from build123d import *

# Parameters (mm, degrees)
F0_W     = 114.3
F0_H     = 330.2
F1_DEPTH = 5.842
F2_W     = 38.1
F2_H     = 5.842
F2_W_2   = 5.842
F2_H_2   = 25.4
F3_DEPTH = 25.4
F4_R     = 9.525
F5_DEPTH = 5.842


# Not quite as in the source:
# - a feature names something its author has since deleted; it is built from what else it names


with BuildPart() as f1:
    # F0 (on Front) → F1 (new body)
    with BuildSketch(Plane.XZ):
        with Locations((-25.4490938969, 91.3394362139)):
            Rectangle(F0_W, F0_H)
    extrude(amount=F1_DEPTH)

    # F2 (on face) → F3 (cut)
    with BuildSketch(Plane.XZ.offset(5.842)):
        Polygon((-82.5990938969, -73.7605637861), (-69.8990938969, -73.7605637861), (-69.8990938969, -67.9185637861), (-76.7570938969, -67.9185637861), (-76.7570938969, -48.3605637861), (-82.5990938969, -48.3605637861), align=None)
        with Locations((-25.4490938969, -70.8395637861)):
            Rectangle(F2_W, F2_H)
        Polygon((19.0009061031, -67.9185637861), (19.0009061031, -73.7605637861), (31.7009061031, -73.7605637861), (31.7009061031, -48.3605637861), (25.8589061031, -48.3605637861), (25.8589061031, -67.9185637861), align=None)
        with Locations((-79.6780938969, -10.2605637861)):
            Rectangle(F2_W_2, F2_H_2)
        with Locations((28.7799061031, -10.2605637861)):
            Rectangle(F2_W_2, F2_H_2)
        with Locations((-79.6780938969, 40.5394362139)):
            Rectangle(F2_W_2, F2_H_2)
        with Locations((28.7799061031, 40.5394362139)):
            Rectangle(F2_W_2, F2_H_2)
        with Locations((-79.6780938969, 91.3394362139)):
            Rectangle(F2_W_2, F2_H_2)
        with Locations((28.7799061031, 91.3394362139)):
            Rectangle(F2_W_2, F2_H_2)
        with Locations((-79.6780938969, 142.1394362139)):
            Rectangle(F2_W_2, F2_H_2)
        with Locations((28.7799061031, 142.1394362139)):
            Rectangle(F2_W_2, F2_H_2)
        with Locations((-79.6780938969, 192.9394362139)):
            Rectangle(F2_W_2, F2_H_2)
        with Locations((28.7799061031, 192.9394362139)):
            Rectangle(F2_W_2, F2_H_2)
        with Locations((28.7799061031, 243.7394362139)):
            Rectangle(F2_W_2, F2_H_2)
        with Locations((-79.6780938969, 243.7394362139)):
            Rectangle(F2_W_2, F2_H_2)
    extrude(amount=-F3_DEPTH, mode=Mode.SUBTRACT)

    # F4 (on face) → F5 (cut, through all)
    with BuildSketch(Plane.XZ.offset(5.842)):
        with BuildLine():
            ThreePointArc((-11.7009406501, 159.6019361475), (-10.1150214145, 163.4306838358), (-9.5740938969, 167.5394362139))
            ThreePointArc((-9.5740938969, 167.5394362139), (-10.1150214004, 171.6481885393), (-11.7009405957, 175.4769361859))
            ThreePointArc((-11.7009405957, 175.4769361859), (-17.5115938829, 181.2875894909), (-25.4490938969, 183.4144362139))
            ThreePointArc((-25.4490938969, 183.4144362139), (-33.3865937403, 181.2875895894), (-39.1972470011, 175.4769365272))
            ThreePointArc((-39.1972470011, 175.4769365272), (-41.3240938969, 167.5394362139), (-39.1972470011, 159.6019359006))
            ThreePointArc((-39.1972470011, 159.6019359006), (-33.3865937403, 153.7912828383), (-25.4490938969, 151.6644362139))
            ThreePointArc((-25.4490938969, 151.6644362139), (-17.5115939301, 153.7912829096), (-11.7009406501, 159.6019361475))
        make_face()
        with Locations((-57.1990938969, 243.7394362139)):
            Circle(F4_R)
        with Locations((6.3009061031, 243.7394362139)):
            Circle(F4_R)
        Polygon((-32.5182228501, 91.3394362139), (-41.6836583735, 107.2144362139), (-60.0145294203, 107.2144362139), (-69.1799649437, 91.3394362139), (-60.0145294203, 75.4644362139), (-41.6836583735, 75.4644362139), align=None)
        Polygon((18.2817771499, 91.3394362139), (9.1163416265, 107.2144362139), (-9.2145294203, 107.2144362139), (-18.3799649437, 91.3394362139), (-9.2145294203, 75.4644362139), (9.1163416265, 75.4644362139), align=None)
        with BuildLine():
            ThreePointArc((-39.1972470011, 175.4769365272), (-33.3865937403, 181.2875895894), (-25.4490938969, 183.4144362139))
            Line((-25.4490938969, 183.4144362139), (-34.6145294203, 183.4144362139))
            Line((-34.6145294203, 183.4144362139), (-39.1972470011, 175.4769365272))
        make_face()
        with BuildLine():
            ThreePointArc((-25.4490938969, 183.4144362139), (-17.5115938829, 181.2875894909), (-11.7009405957, 175.4769361859))
            Line((-11.7009405957, 175.4769361859), (-16.2836583735, 183.4144362139))
            Line((-16.2836583735, 183.4144362139), (-25.4490938969, 183.4144362139))
        make_face()
        with BuildLine():
            ThreePointArc((-11.7009405957, 175.4769361859), (-10.1150214004, 171.6481885393), (-9.5740938969, 167.5394362139))
            ThreePointArc((-9.5740938969, 167.5394362139), (-10.1150214145, 163.4306838358), (-11.7009406501, 159.6019361475))
            Line((-11.7009406501, 159.6019361475), (-7.1182228501, 167.5394362139))
            Line((-7.1182228501, 167.5394362139), (-11.7009405957, 175.4769361859))
        make_face()
        with BuildLine():
            Line((-16.2836583735, 151.6644362139), (-11.7009406501, 159.6019361475))
            ThreePointArc((-11.7009406501, 159.6019361475), (-17.5115939301, 153.7912829096), (-25.4490938969, 151.6644362139))
            Line((-25.4490938969, 151.6644362139), (-16.2836583735, 151.6644362139))
        make_face()
        with BuildLine():
            Line((-34.6145294203, 151.6644362139), (-25.4490938969, 151.6644362139))
            ThreePointArc((-25.4490938969, 151.6644362139), (-33.3865937403, 153.7912828383), (-39.1972470011, 159.6019359006))
            Line((-39.1972470011, 159.6019359006), (-34.6145294203, 151.6644362139))
        make_face()
        with BuildLine():
            ThreePointArc((-39.1972470011, 159.6019359006), (-41.3240938969, 167.5394362139), (-39.1972470011, 175.4769365272))
            Line((-39.1972470011, 175.4769365272), (-43.7799649437, 167.5394362139))
            Line((-43.7799649437, 167.5394362139), (-39.1972470011, 159.6019359006))
        make_face()
    extrude(amount=-F5_DEPTH, mode=Mode.SUBTRACT)


solid = f1.part
Geometry check sheet. Reference: the model listing, model coordinates, mm. A direction names the side the tool comes from. Round coordinates to 2 decimals unless told otherwise and drop trailing zeros. Write each loop counter-clockwise with the first axis right and the second up, starting at its lowest first coordinate (ties: lowest second). Pieces come first, ordered by that corner, then holes. Notation, with made-up numbers: (-0.5, -8.75) - (50.5, -8.75) arc R30 cw to (50.5, 28.25) - close; hole circle Ø5 at (-20, 1). An arc over 180 degrees is marked (long way). One line per item, written item: value.
1. Cross-section at C-C on z = 163. Record the boundary of the cut face in (x, y), and give its area (3 significant figures).
The answers:
outline: (-82.6, -5.84) - (-41.16, -5.84) - (-41.16, 0) - (-82.6, 0) - close; (-9.74, -5.84) - (31.7, -5.84) - (31.7, 0) - (-9.74, 0) - close
area: 484 mm^2
2. Depth check by flat-ended pin: pin 1 Ø3 at (x, y) = (-80, -4) entering from +Z; pin 2 Ø1.8 at (x, y) = (-21.5, -3.5) entering from -Z; pin 3 Ø3 at (y, z) = (-3.5, -11) entering from -X. Enter the tip coordinate at first touch or a pass-through.
The answers:
pin 1: stops at z = 231.04
pin 2: stops at z = -67.92
pin 3: stops at x = -76.76
3. Cross-section at B-B on z = 85. Record the boundary of the cut face in (x, y).
The answers:
outline: (-76.76, -5.84) - (-65.52, -5.84) - (-65.52, 0) - (-76.76, 0) - close; (-36.18, -5.84) - (-14.72, -5.84) - (-14.72, 0) - (-36.18, 0) - close; (14.62, -5.84) - (25.86, -5.84) - (25.86, 0) - (14.62, 0) - close
4. Mould release check, pull along Z, two halves, no side actions. Record for faces 1 (the face through (6, -3, -73.761)), 2 (the face through (31.701, -3, -36)), 3 (the face through (-64.53, -2.96, 99.39)), 4 (the face through (29, -3, 231.039)): released by +Z, released by -Z, zero draft, split by the parting line, or undercut.
The answers:
face 1: released by -Z
face 2: zero draft
face 3: undercut
face 4: released by +Z
5. Scan lines: L1, parallel to Z at x = -57, y = -1.1; L2, parallel to Z at x = -60, y = -2.05; L3, parallel to Z at x = -3.5, y = -4.85. Record each from-to range of solid material in increasing order.
The answers:
L1: z = -73.76 to 75.46, 107.21 to 234.22, 253.26 to 256.44
L2: z = -73.76 to 75.46, 107.21 to 234.64, 252.84 to 256.44
L3: z = -73.76 to 75.46, 107.21 to 256.44
6. Cross-section at D-D on x = -73.5. Record the boundary of the cut face in (y, z).
The answers:
outline: (-5.84, -67.92) - (0, -67.92) - (0, 256.44) - (-5.84, 256.44) - close
7. Set-up check for faces 5 (the face through (25.859, -3, 244)), 6 (the face through (-76.757, -3, 244)), 7 (the face through (13.76, -2.96, 99.17)), 8 (the face through (25.859, -3, -10)): record each of +Z, -Z, +X, -X, +Y, -Y from which the full face is reachable in a straight line by a thin tool's end or side.
The answers:
face 5: +Z, +X, +Y, -Y
face 6: +Z, -X, +Y, -Y
face 7: +Y, -Y
face 8: +X, +Y, -Y
8. Cross-section at A-A on x = -25. Record the boundary of the cut face in (y, z).
The answers:
outline: (-5.84, -67.92) - (0, -67.92) - (0, 151.66) - (-5.84, 151.66) - close; (-5.84, 183.41) - (0, 183.41) - (0, 256.44) - (-5.84, 256.44) - close
